Here's how the part is built. I have some questions about the finished solid (model axes, mm). A direction names the side the tool comes from. Give positions to 0.01 mm unless a question says otherwise; leave off trailing zeros. Loops run counter-clockwise (first coordinate to the right, second up) from the corner with the lowest first, then second, coordinate; pieces in that order, holes last.
Q1. Will these pins go through, and if not, where does the flat tip stop? P1, Ø10, axis at y = 16.5, z = -6.5, coming from the -X side; P2, Ø1.5, axis at x = 8, z = -6.5, coming from the +Y side; P3, Ø3.5, axis at x = -23.82, z = -5.5, coming from the -Y side; P4, Ø4, axis at y = 7.5, z = 5.5, coming from the +X side.
Q2. If we section it at D-D (y = 10.5): Please give me the cut outline in (x, z).
Q3. If we section it at A-A (x = -13): Please give me the cut outline in (y, z), plus the area to 3 significant figures.
Q4. If we section it at B-B (z = -5.5): Please give me the cut outline in (x, y), plus the area to 3 significant figures.
Q5. If we section it at C-C (x = 24): Please give me the cut outline in (y, z), plus the area to 3 significant figures.
Q6. We'd pull the mould along X, two halves only. Please class faces 5 (the face through (21.441, 28.014, -3.675)), 6 (the face through (20, 34, 0)), 7 (the face through (-28, 28, 0)), 8 (the face through (24, 27, 0)): +X half, -X half, draft (parallel to the pull), parting line (faces both ways), or undercut.
Q7. For faces 1 (the face through (-20, 34, 0)), 2 (the face through (20, 13, 0)), 3 (the face through (21.611, 28.014, 3.472)), 4 (the face through (-24, 27, 0)), which set-ups out of +Z, -Z, +X, -X, +Y, -Y let a thin tool reach every point of the face, with its end or its side?
Q8. I need wall thicknesses on line 1 (X direction, y = 27.5, z = 5.5); line 2 (Y direction, x = 2, z = -2.5); line 3 (X direction, y = 39, z = -0.25). Which ranges of each line are inside material? Lowest first, please.
from build123d import *

# Parameters (mm, degrees)
SKETCH1_W           = 40
SKETCH1_H           = 20
BOSS_EXTRUDE1_DEPTH = 40
SKETCH2_R           = 3
BOSS_EXTRUDE2_DEPTH = 4
SKETCH3_W           = 20
SKETCH3_H           = 2
BOSS_EXTRUDE3_DEPTH = 8
SKETCH4_R           = 3
CUT_EXTRUDE1_DEPTH  = 30


with BuildPart() as part:
    # Sketch1 → Boss-Extrude1 (new body)
    with BuildSketch(Plane(origin=(0, 0, 0), x_dir=(1, 0, 0), z_dir=(0, 1, 0))):
        Rectangle(SKETCH1_W, SKETCH1_H)
    extrude(amount=BOSS_EXTRUDE1_DEPTH)

    # Sketch2 → Boss-Extrude2 (add)
    with BuildSketch(Plane(origin=(0, 40, 0), x_dir=(1, 0, 0), z_dir=(0, 1, 0))):
        with Locations((-13, 0)):
            Circle(SKETCH2_R)
    extrude(amount=BOSS_EXTRUDE2_DEPTH)

    # Sketch3 → Boss-Extrude3 (add)
    with BuildSketch(Plane(origin=(20, 0, 0), x_dir=(0, 0, -1), z_dir=(1, 0, 0))):
        with Locations((0, 28)):
            Rectangle(SKETCH3_W, SKETCH3_H)
    boss_extrude3 = extrude(amount=BOSS_EXTRUDE3_DEPTH)

    # Sketch4 → Cut-Extrude1 (cut, through all)
    with BuildSketch(Plane(origin=(0, 29, 0), x_dir=(1, 0, 0), z_dir=(0, 1, 0))):
        with Locations((23.821894681, 5.5)):
            Circle(SKETCH4_R)
        with Locations((23.821894681, -5.5)):
            Circle(SKETCH4_R)
    cut_extrude1 = extrude(amount=-CUT_EXTRUDE1_DEPTH, mode=Mode.SUBTRACT)

    # Mirror2: Boss-Extrude3, Cut-Extrude1 across plane
    add(boss_extrude3.mirror(Plane(origin=(0, 0, 0), x_dir=(0, 0, 1), z_dir=(1, 0, 0))))
    add(cut_extrude1.mirror(Plane(origin=(0, 0, 0), x_dir=(0, 0, 1), z_dir=(1, 0, 0))), mode=Mode.SUBTRACT)


solid = part.part
Check sheet entries:
1. P1: stops at x = -20
1. P2: stops at y = 40
1. P3: passes through
1. P4: stops at x = 20
2. outline: (-20, -10) - (20, -10) - (20, 10) - (-20, 10) - close
3. outline: (0, -10) - (40, -10) - (40, -3) - (44, -3) - (44, 3) - (40, 3) - (40, 10) - (0, 10) - close
3. area: 824 mm2
4. outline: (-28, 27) - (-26.82, 27) - (-26.82, 29) - (-28, 29) - close; (-20.82, 27) - (-20, 27) - (-20, 0) - (20, 0) - (20, 27) - (20.82, 27) - (20.82, 29) - (20, 29) - (20, 40) - (-20, 40) - (-20, 29) - (-20.82, 29) - close; (26.82, 27) - (28, 27) - (28, 29) - (26.82, 29) - close
4. area: 1,610 mm2
5. outline: (27, -10) - (29, -10) - (29, -8.49) - (27, -8.49) - close; (27, -2.51) - (29, -2.51) - (29, 2.51) - (27, 2.51) - close; (27, 8.49) - (29, 8.49) - (29, 10) - (27, 10) - close
5. area: 16.0 mm2
6. face 5: undercut
6. face 6: +X half
6. face 7: -X half
6. face 8: draft
7. face 1: +Z, -Z, -X, +Y
7. face 2: +Z, -Z, +X, -Y
7. face 3: +Y, -Y
7. face 4: +Z, -Z, -X, -Y
8. line 1: x = -28 to -26.82, -20.82 to 20.82, 26.82 to 28
8. line 2: y = 0 to 40
8. line 3: x = -20 to 20
